Work out the finished part from the listing and answer in its coordinate system (mm). Face numbers are marked on the shaded views. Round coordinates to 2 decimals unless told otherwise and drop trailing zeros. Order: outer loops, then holes, each group sorted by start corner. A loop starts at its lowest first (then second) coordinate and runs counter-clockwise, first axis right, second up. Notation, with made-up numbers: (73.5, 3) -> (105.5, 3) arc R37 cw to (105.5, 41) -> close; hole circle Ø1 at (-26, -32). An arc over 180 degrees is marked (long way). Use a Markdown table: item, result. Add a question column.
Item 1: Flat-ended cylindrical pins translate along their axes: P1, Ø0.6, axis at y = 3, z = -81, coming from the +X side; P2, Ø1.6, axis at y = 42, z = -83, coming from the +X side; P3, Ø2, axis at y = 47.5, z = -83.5, coming from the -X side; P4, Ø8, axis at x = -164, y = 36, coming from the -Z side. Find the tip coordinate at first contact, or state that the pin passes through.
Item 2: For a pull along Y with two mould halves and no side action, classify the marked faces 1, 2 and 3 as +Y half, -Y half, draft (parallel to the pull), parting line (faces both ways), or undercut.
Item 3: A cutting plane is placed at B-B, the plane z = -70.5. Determine the outline of the cut face in (x, y), plus the area to 3 significant figures.
Item 4: A cutting plane is placed at A-A, the plane y = 52. Determine the outline of the cut face in (x, z).
Item 5: A cutting plane is placed at D-D, the plane x = -175.5. Determine the outline of the cut face in (y, z).
Item 6: A cutting plane is placed at C-C, the plane y = 12. Determine the outline of the cut face in (x, z), plus the area to 3 significant figures.
Item 7: Find the intervals of material crossed by L1, parallel to Y at x = -138, z = -82.5; L2, parallel to Y at x = -125, z = -79.25; L3, parallel to Z at x = -150, y = 34.5, in increasing order. Write a range as [from, to].
from build123d import *

# Parameters (mm, degrees)
SKETCH1_W           = 92.6
SKETCH1_H           = 22
BOSS_EXTRUDE1_DEPTH = 2
FILLET1_R           = 2
SKETCH5_W           = 20.6
SKETCH5_H           = 2
BOSS_EXTRUDE3_DEPTH = 60
SKETCH6_W           = 6
SKETCH6_H           = 2
BOSS_EXTRUDE4_DEPTH = 4
SKETCH7_R           = 2.3
CUT_EXTRUDE1_DEPTH  = 2
FILLET4_R           = 30


with BuildPart() as part:
    # Sketch1 → Boss-Extrude1 (new body)
    with BuildSketch(Plane(origin=(0, 0, 0), x_dir=(1, 0, 0), z_dir=(0, 1, 0))):
        with Locations((-146.346488806, 73.566618989)):
            Rectangle(SKETCH1_W, SKETCH1_H)
    extrude(amount=BOSS_EXTRUDE1_DEPTH)

    # Fillet1
    fillet1_edges = [part.edges().sort_by_distance(p)[0] for p in [
        (-100.046488806, 1, -62.566618989),
        (-192.646488806, 1, -62.566618989),
    ]]
    fillet(fillet1_edges, radius=FILLET1_R)

    # Sketch5 → Boss-Extrude3 (add)
    with BuildSketch(Plane(origin=(0, 2, 0), x_dir=(1, 0, 0), z_dir=(0, 1, 0))):
        with Locations((-146.346488806, 83.566618989)):
            Rectangle(SKETCH5_W, SKETCH5_H)
    extrude(amount=BOSS_EXTRUDE3_DEPTH)

    # Sketch6 → Boss-Extrude4 (add)
    with BuildSketch(Plane.XY.offset(-82.566618989)):
        with Locations((-151.546488806, 61)):
            Rectangle(SKETCH6_W, SKETCH6_H)
        with Locations((-140.546488806, 61)):
            Rectangle(SKETCH6_W, SKETCH6_H)
        with Locations((-152.046488806, 3)):
            Rectangle(SKETCH6_W, SKETCH6_H)
        with Locations((-141.046488806, 3)):
            Rectangle(SKETCH6_W, SKETCH6_H)
    extrude(amount=BOSS_EXTRUDE4_DEPTH)

    # Sketch7 → Cut-Extrude1 (cut)
    with BuildSketch(Plane.XY.offset(-82.566618989)):
        with Locations((-146.046488806, 52)):
            Circle(SKETCH7_R)
        with Locations((-146.046488806, 12)):
            Circle(SKETCH7_R)
    extrude(amount=-CUT_EXTRUDE1_DEPTH, mode=Mode.SUBTRACT)

    # Fillet4
    fillet4_edges = [part.edges().sort_by_distance(p)[0] for p in [
        (-156.646488806, 2, -83.566618989),
        (-136.046488806, 2, -83.566618989),
    ]]
    fillet(fillet4_edges, radius=FILLET4_R)


solid = part.part
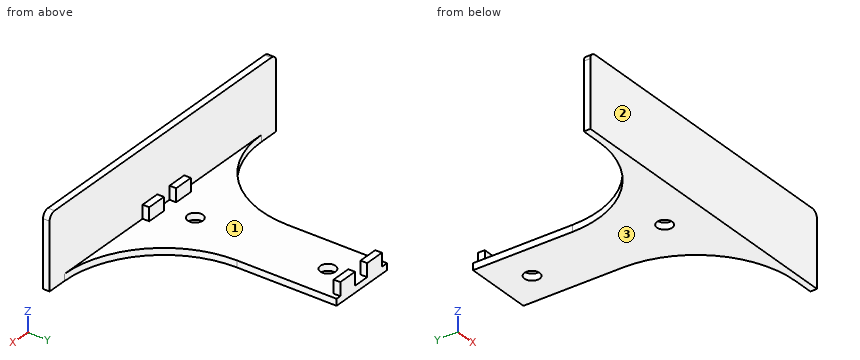
Reported:
| question | item | result |
|---|---|---|
| 1 | P1 | x = -138.05 |
| 1 | P2 | x = -136.05 |
| 1 | P3 | x = -156.65 |
| 1 | P4 | through |
| 2 | face 1 | undercut |
| 2 | face 2 | -Y half |
| 2 | face 3 | draft |
| 3 | outline | (-192.65, 0) -> (-100.05, 0) -> (-100.05, 2) -> (-192.65, 2) -> close |
| 3 | area | 185 mm² |
| 4 | outline | (-156.65, -84.57) -> (-148.35, -84.57) -> (-148.35, -82.57) -> (-156.65, -82.57) -> close; (-143.75, -84.57) -> (-136.05, -84.57) -> (-136.05, -82.57) -> (-143.75, -82.57) -> close |
| 5 | outline | (0, -84.57) -> (4.15, -84.57) -> (4.15, -82.57) -> (2, -82.57) -> (2, -62.57) -> (0, -62.57) -> close |
| 6 | outline | (-164.29, -84.57) -> (-148.35, -84.57) -> (-148.35, -82.57) -> (-164.29, -82.57) -> close; (-143.75, -84.57) -> (-128.41, -84.57) -> (-128.41, -82.57) -> (-143.75, -82.57) -> close |
| 6 | area | 62.6 mm² |
| 7 | L1 | [0, 2], [60, 62] |
| 7 | L2 | [0, 2] |
| 7 | L3 | [-84.57, -82.57] |
